The listing builds one solid part. Answer for the finished solid, in the listing's coordinates (mm). Face numbers are marked on the shaded views. A direction names the side the tool comes from. Give positions to 0.01 mm unless a question says otherwise; leave off trailing zeros. Write each loop counter-clockwise with the first axis right and the second up, starting at its lowest first coordinate (ties: lowest second). Pieces come first, ordered by that corner, then holes. Notation, with made-up numbers: (-29.75, 0) -> (12.25, 0) arc R23 cw to (12.25, 14) -> close; hole circle Ø6 at (-14.5, 29.25). An arc over 180 degrees is marked (long way). One line per question, with ' | ' between items.
from build123d import *

# Parameters (mm, degrees)
SKETCH2_R           = 5.0419
SKETCH2_R_2         = 2.0574
BOSS_EXTRUDE1_DEPTH = 19.05
BOSS_EXTRUDE2_DEPTH = 19.05
SKETCH3_R           = 2.4384
CUT_EXTRUDE1_DEPTH  = 12.7
SKETCH4_W           = 1.27
SKETCH4_H           = 6.35
CUT_EXTRUDE2_DEPTH  = 22.060567509


with BuildPart() as part:
    # Sketch2 → Boss-Extrude1 (new body)
    with BuildSketch(Plane.XY):
        with Locations(Location((0, 0, 0), (0, 0, 180))):
            Circle(SKETCH2_R)
        with Locations(Location((0, 0, 0), (0, 0, 180))):
            Circle(SKETCH2_R_2, mode=Mode.SUBTRACT)
    extrude(amount=BOSS_EXTRUDE1_DEPTH)

    # Sketch6 → Boss-Extrude2 (add)
    with BuildSketch(Plane(origin=(0, 0, 0), x_dir=(-1, 0, 0), z_dir=(0, 0, -1))):
        with BuildLine():
            Line((1.461769448, 1.4478), (-1.461769448, 1.4478))
            ThreePointArc((-1.461769448, 1.4478), (0, 2.0574), (1.461769448, 1.4478))
        make_face()
    extrude(amount=-BOSS_EXTRUDE2_DEPTH)

    # Sketch3 → Cut-Extrude1 (cut, symmetric)
    with BuildSketch(Plane.XZ):
        with Locations(Location((0, 14.732, 0), (0, 0, 270))):
            Circle(SKETCH3_R)
    extrude(amount=CUT_EXTRUDE1_DEPTH, both=True, mode=Mode.SUBTRACT)

    # Sketch4 → Revolve1 (revolve)
    with BuildSketch(Plane(origin=(0, 0, 0), x_dir=(0, 0, -1), z_dir=(1, 0, 0)), mode=Mode.PRIVATE) as revolve1_sk:
        with Locations((-19.685, 3.175)):
            Rectangle(SKETCH4_W, SKETCH4_H)
    revolve(revolve1_sk.sketch.rotate(Axis((0, 0, 0), (0, 0, -1)), 90), axis=Axis((0, 0, 0), (0, 0, -1)))

    # Sketch5 → Cut-Extrude2 (cut, through all)
    with BuildSketch(Plane(origin=(0, 0, 19.05), x_dir=(-1, 0, 0), z_dir=(0, 0, -1))):
        with BuildLine():
            Line((1.461769448, 1.4478), (-1.461769448, 1.4478))
            ThreePointArc((-1.461769448, 1.4478), (0, -2.0574), (1.461769448, 1.4478))
        make_face()
    extrude(amount=-CUT_EXTRUDE2_DEPTH, mode=Mode.SUBTRACT)


solid = part.part
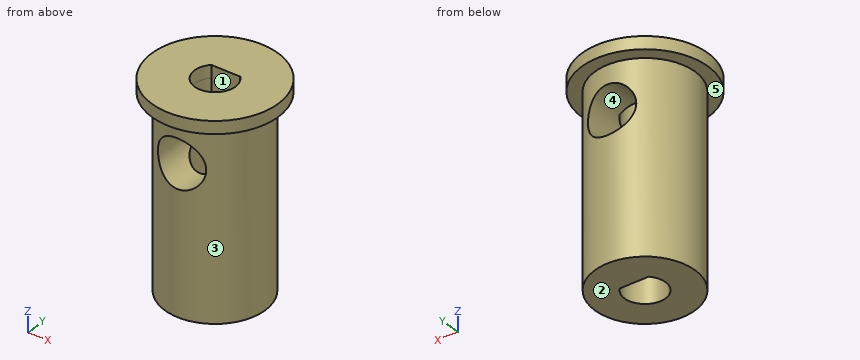
Item 1: A tool of negligible diameter and unlimited length cuts with its end or side. For the marked faces 4 and 5, from which of +Z, -Z, +X, -X, +Y, -Y can it reach the whole face along a straight path? Write none if from no direction.
Answers below:
face 4: +Y, -Y | face 5: -Z
Item 2: Find section B-B (y = 0). Write down the section's boundary in (x, z).
Answers below:
outline: (-6.35, 19.05) -> (-5.04, 19.05) -> (-5.04, 0) -> (-2.06, 0) -> (-2.06, 13.42) arc R2.44 cw to (-2.06, 16.04) -> (-2.06, 20.32) -> (-6.35, 20.32) -> close; (2.06, 0) -> (5.04, 0) -> (5.04, 19.05) -> (6.35, 19.05) -> (6.35, 20.32) -> (2.06, 20.32) -> (2.06, 16.04) arc R2.44 cw to (2.06, 13.42) -> close
Item 3: Find section C-C (z = 13). Write down the section's boundary in (x, y), then the cut area to 3 significant figures.
Answers below:
outline: (-1.72, -4.74) -> (-1.72, -1.13) arc R2.06 cw to (-1.72, 1.13) -> (-1.72, 4.74) arc R5.04 ccw to start; (1.72, -4.74) arc R5.04 ccw to (1.72, 4.74) -> (1.72, 1.13) arc R2.06 cw to (1.72, -1.13) -> close | area: 44.9 mm²
Item 4: Find section A-A (x = 0). Write down the section's boundary in (y, z), then the cut area to 3 significant figures.
Answers below:
outline: (-6.35, 19.05) -> (-5.04, 19.05) -> (-5.04, 17.17) -> (-2.06, 17.17) -> (-2.06, 20.32) -> (-6.35, 20.32) -> close; (-5.04, 0) -> (-2.06, 0) -> (-2.06, 12.29) -> (-5.04, 12.29) -> close; (1.45, 0) -> (5.04, 0) -> (5.04, 12.29) -> (1.45, 12.29) -> close; (1.45, 17.17) -> (5.04, 17.17) -> (5.04, 19.05) -> (6.35, 19.05) -> (6.35, 20.32) -> (1.45, 20.32) -> close | area: 105 mm²
Item 5: Find section D-D (y = 3.5). Write down the section's boundary in (x, z), then the cut area to 3 significant figures.
Answers below:
outline: (-5.3, 19.05) -> (-3.63, 19.05) -> (-3.63, 0) -> (3.63, 0) -> (3.63, 19.05) -> (5.3, 19.05) -> (5.3, 20.32) -> (-5.3, 20.32) -> close; hole circle Ø4.88 at (0, 14.73) | area: 133 mm²
Item 6: Flat-ended cylindrical pins translate along their axes: pin 1 (1.5 mm diameter, centred on x = 0.5, z = 5.5, fed in from -Y); pin 2 (4 mm diameter, centred on x = 3, z = 10.5, fed in from +Y); pin 3 (5.5 mm diameter, centred on x = 0, z = 14.732, fed in from +Y). Find the tip coordinate at first contact, or state that the pin passes through.
Answers below:
pin 1: y = -5.04 | pin 2: y = 4.94 | pin 3: y = 5.04
Item 7: Consider line 1 (Y direction, x = 0, z = 8.75); line 2 (Z direction, x = 0, y = -3); line 3 (Z direction, x = -4.5, y = 2.75). Determine where each line is inside the solid, lowest interval first. Write a range as [from, to].
Answers below:
line 1: [-5.04, -2.06], [1.45, 5.04] | line 2: [0, 12.29], [17.17, 20.32] | line 3: [19.05, 20.32]
Item 8: Determine the mould class of the marked faces 1, 2 and 3 for opening direction Y: pulls with the +Y half, pulls with the -Y half, needs draft (parallel to the pull), parting line crosses it, or undercut.
Answers below:
face 1: undercut | face 2: needs draft | face 3: parting line crosses it
